from build123d import *

# Parameters (mm, degrees)
SKETCH1_W           = 29
SKETCH1_H           = 17
SKETCH1_R           = 1.5
BOSS_EXTRUDE1_DEPTH = 3
SKETCH1_3_W         = 29
SKETCH1_3_H         = 17
SKETCH1_3_W_2       = 27
SKETCH1_3_H_2       = 15
BOSS_EXTRUDE2_DEPTH = 0.5
SKETCH3_W           = 19
SKETCH3_H           = 1
CUT_EXTRUDE1_DEPTH  = 6
BOSS_EXTRUDE3_DEPTH = 3
BOSS_EXTRUDE4_DEPTH = 1.5


with BuildPart() as part:
    # Sketch1 → Boss-Extrude1 (new body)
    with BuildSketch(Plane(origin=(0, 0, 0), x_dir=(1, 0, 0), z_dir=(0, 1, 0))):
        Rectangle(SKETCH1_W, SKETCH1_H)
        with Locations((-9, 5.5)):
            Circle(SKETCH1_R, mode=Mode.SUBTRACT)
        with Locations((9, 5.5)):
            Circle(SKETCH1_R, mode=Mode.SUBTRACT)
        with Locations((-6, -5.5)):
            Circle(SKETCH1_R, mode=Mode.SUBTRACT)
        with Locations((6, -5.5)):
            Circle(SKETCH1_R, mode=Mode.SUBTRACT)
    extrude(amount=BOSS_EXTRUDE1_DEPTH)

    # Sketch1_3 → Boss-Extrude2 (add)
    with BuildSketch(Plane(origin=(0, 0, 0), x_dir=(1, 0, 0), z_dir=(0, 1, 0))):
        Rectangle(SKETCH1_3_W, SKETCH1_3_H)
        Rectangle(SKETCH1_3_W_2, SKETCH1_3_H_2, mode=Mode.SUBTRACT)
    extrude(amount=-BOSS_EXTRUDE2_DEPTH)

    # Sketch3 → Cut-Extrude1 (cut)
    with BuildSketch(Plane.XY.offset(8.5)):
        with Locations((0, -0.5)):
            Rectangle(SKETCH3_W, SKETCH3_H)
    extrude(amount=-CUT_EXTRUDE1_DEPTH, mode=Mode.SUBTRACT)

    # Sketch4 → Boss-Extrude3 (add, symmetric)
    with BuildSketch(Plane.XY):
        with BuildLine():
            Line((-10.638572491, 3), (-9.176228871, 3))
            ThreePointArc((-9.176228871, 3), (-6.583274937, 8.845404617), (-6.076469935, 15.219988049))
            Line((-6.076469935, 15.219988049), (-10.638572491, 19.393054364))
            Line((-10.638572491, 19.393054364), (-10.638572491, 3))
        make_face()
        with BuildLine():
            Line((-65, -5.482953492), (-25, -5.482953492))
            ThreePointArc((-25, -5.482953492), (-19.516691912, -4.674526607), (-14.5, -2.318041114))
            Line((-14.5, -2.318041114), (-14.5, 3))
            Line((-14.5, 3), (-10.638572491, 3))
            Line((-10.638572491, 3), (-10.638572491, 19.393054364))
            Line((-10.638572491, 19.393054364), (-6.076469935, 15.219988049))
            ThreePointArc((-6.076469935, 15.219988049), (-7.534123574, 20.996562579), (-10.709024477, 26.037750106))
            Line((-10.709024477, 26.037750106), (-13.79929628, 28.864496986))
            ThreePointArc((-13.79929628, 28.864496986), (-19.109395578, 31.580843992), (-25, 32.517046508))
            Line((-25, 32.517046508), (-65, 32.517046508))
            ThreePointArc((-65, 32.517046508), (-84, 13.517046508), (-65, -5.482953492))
        make_face()
        with BuildLine():
            ThreePointArc((-25, 22.517046508), (-16, 13.517046508), (-25, 4.517046508))
            Line((-25, 4.517046508), (-65, 4.517046508))
            ThreePointArc((-65, 4.517046508), (-74, 13.517046508), (-65, 22.517046508))
            Line((-65, 22.517046508), (-25, 22.517046508))
        make_face(mode=Mode.SUBTRACT)
        with BuildLine():
            Line((-6.076469935, 15.219988049), (7.282732748, 3))
            Line((7.282732748, 3), (14.476431663, 3))
            Line((14.476431663, 3), (-10.709024477, 26.037750106))
            ThreePointArc((-10.709024477, 26.037750106), (-7.534123574, 20.996562579), (-6.076469935, 15.219988049))
        make_face()
    extrude(amount=BOSS_EXTRUDE3_DEPTH, both=True)

    # Sketch4_3 → Boss-Extrude4 (add, symmetric)
    with BuildSketch(Plane.XY):
        with BuildLine():
            ThreePointArc((-6.076469935, 15.219988049), (-6.583274937, 8.845404617), (-9.176228871, 3))
            Line((-9.176228871, 3), (7.282732748, 3))
            Line((7.282732748, 3), (-6.076469935, 15.219988049))
        make_face()
    extrude(amount=BOSS_EXTRUDE4_DEPTH, both=True)


solid = part.part
Design review of the part built by this model. Coordinates are the model's own, in mm. A direction names the side the tool comes from. Round coordinates to 2 decimals unless told otherwise and drop trailing zeros. Write each loop counter-clockwise with the first axis right and the second up, starting at its lowest first coordinate (ties: lowest second). Pieces come first, ordered by that corner, then holes. Notation, with made-up numbers: M 78.25,66 L 90.25,66 A29 ccw 90.25,95 Z; hole C 6.25,-37 d10. An arc over 180 degrees is marked long. One line per item, written item: value. Start each with the question number.
1. Take a section at C-C on x = 6. State the section outline as (y, z) points, then the cut area to 3 significant figures.
2. For faces 5 (the face through (-3, 6, 1.5)), 6 (the face through (-1, -0.5, -8)), 7 (the face through (-73.998, 13.319, 0.042)), list the 3-axis set-ups (+Z, -Z, +X, -X, +Y, -Y) from which the entire face can be reached by the end or side of a thin tool; tool diameter is ignored.
3. To check wall thickness, follow probe 1 along X at (y, z) = (1.4, -5.5); probe 2 along X at (y, z) = (1.45, 5.5); probe 3 along Y at (x, z) = (-44, 0.75). State the ranges of each line that lie inside material, in increasing order. Write a range as from..to.
4. Take a section at A-A on x = -41. State the section outline as (y, z) points, then the cut area to 3 significant figures.
5. Take a section at D-D on y = 24.5. State the section outline as (x, z) points, then the cut area to 3 significant figures.
6. Draft analysis for pull direction Y (two halves, no side actions). For faces 1 (the face through (-45, -5.483, 0)), 2 (the face through (-10.5, 1.48, -5.57)), 3 (the face through (-16, 13.7, 0)), 4 (the face through (-6.606, 8.758, 2.26)), state which applies: pulls with the +Y half, pulls with the -Y half, needs draft (parallel to the pull), parting line crosses it, or undercut.
7. Clearance check with flat-ended pins moving along their axes: P1, Ø2, axis at y = 7.5, z = 3.5, coming from the +X side; P2, Ø8, axis at x = -11.5, y = 7.5, coming from the -Z side; P3, Ø10, axis at x = -0.5, z = 5.5, coming from the +Y side. State where each tip first meets the part, or that it passes through.
Computed:
1. outline: M -0.5,-8.5 L 3,-8.5 L 3,-1.5 L 4.17,-1.5 L 4.17,-3 L 10.75,-3 L 10.75,3 L 4.17,3 L 4.17,1.5 L 3,1.5 L 3,4 L 0,4 L 0,-7.5 L -0.5,-7.5 Z; M 0,7 L 3,7 L 3,8.5 L 0,8.5 Z
1. area: 85.5 mm²
2. face 5: +Z
2. face 6: +Z, -Z, +X, -Y
2. face 7: +Z, -Z
3. probe 1: x = -14.5..-10.5, -7.5..7.5, 10.5..14.5
3. probe 2: x = -14.5..-7.5, -4.5..4.5, 7.5..14.5
3. probe 3: y = -5.48..4.52, 22.52..32.52
4. outline: M -5.48,-3 L 4.52,-3 L 4.52,3 L -5.48,3 Z; M 22.52,-3 L 32.52,-3 L 32.52,3 L 22.52,3 Z
4. area: 120 mm²
5. outline: M -80.5,-3 L -9.03,-3 L -9.03,3 L -80.5,3 Z
5. area: 429 mm²
6. face 1: pulls with the -Y half
6. face 2: needs draft
6. face 3: undercut
6. face 4: undercut
7. P1: stops at x = 10.5
7. P2: stops at z = -3
7. P3: stops at y = 20.66
